from build123d import *

# Parameters (mm, degrees)
SKETCH_2_W                    = 37.5
SKETCH_2_H                    = 19
EXTRUDE_1_DEPTH               = 1.6
SKETCH_3_W                    = 23
SKETCH_3_H                    = 13.4
EXTRUDE_2_DEPTH               = 10.4
FILLET_1_R                    = 2
SKETCH_4_W                    = 4
SKETCH_4_H                    = 3
CUT_EXTRUDE_1_DEPTH           = 1.6
FILLET_2_R                    = 1.5
SKETCH_5_R                    = 1.5
CUT_EXTRUDE_2_DEPTH           = 5
SKETCH_6_W                    = 8
SKETCH_6_H                    = 6
CUT_EXTRUDE_3_DEPTH           = 1
CUT_EXTRUDE_3_DRAFT           = -57
CUT_EXTRUDE_3_PROFILE_2_DEPTH = 1
CUT_EXTRUDE_3_PROFILE_2_DRAFT = -57
FILLET_3_R                    = 5.5
SKETCH_7_W                    = 8
SKETCH_7_H                    = 7
EXTRUDE_3_DEPTH               = 1
SKETCH_8_W                    = 8
SKETCH_8_H                    = 3.15
SKETCH_8_H_2                  = 3.13772234
EXTRUDE_4_DEPTH               = 1
FILLET_4_R                    = 2
SKETCH_9_W                    = 3
SKETCH_9_H                    = 0.2
EXTRUDE_5_DEPTH               = 2
SKETCH_10_W                   = 3
SKETCH_10_H                   = 7
EXTRUDE_6_DEPTH               = 0.2
SKETCH_11_W                   = 1.5
SKETCH_11_H                   = 3
CUT_EXTRUDE_4_DEPTH           = 0.2
FILLET_5_R                    = 0.75


# Some blends are built 0.0001 mm under size
with BuildPart() as part:
    # Эскиз2 → Бобышка-Вытянуть1 (new body)
    with BuildSketch(Plane.XY):
        Rectangle(SKETCH_2_W, SKETCH_2_H)
    extrude(amount=EXTRUDE_1_DEPTH)

    # Эскиз3 → Бобышка-Вытянуть2 (add)
    with BuildSketch(Plane.XY.offset(1.6)):
        Rectangle(SKETCH_3_W, SKETCH_3_H)
    extrude(amount=EXTRUDE_2_DEPTH)

    # Скругление1
    fillet_1_edges = [part.edges().sort_by_distance(p)[0] for p in [
        (-18.75, 9.5, 0.8),
        (18.75, 9.5, 0.8),
        (18.75, -9.5, 0.8),
        (-18.75, -9.5, 0.8),
    ]]
    fillet(fillet_1_edges, radius=FILLET_1_R)

    # Эскиз4 → Вырез-Вытянуть1 (cut)
    with BuildSketch(Plane.XY.offset(1.6)):
        with Locations((14.75, 0)):
            Rectangle(SKETCH_4_W, SKETCH_4_H)
        with Locations((-14.75, 0)):
            Rectangle(SKETCH_4_W, SKETCH_4_H)
    extrude(amount=-CUT_EXTRUDE_1_DEPTH, mode=Mode.SUBTRACT)

    # Скругление2
    fillet_2_edges = [part.edges().sort_by_distance(p)[0] for p in [
        (-16.75, 1.5, 0.8),
        (-12.75, 1.5, 0.8),
        (16.75, 1.5, 0.8),
        (16.75, -1.5, 0.8),
        (-12.75, -1.5, 0.8),
        (-16.75, -1.5, 0.8),
        (12.75, -1.5, 0.8),
        (12.75, 1.5, 0.8),
    ]]
    fillet(fillet_2_edges, radius=FILLET_2_R - 0.0001)  # a hair under: the kernel refuses the full size

    # Эскиз5 → Вырез-Вытянуть2 (cut)
    with BuildSketch(Plane.XY.offset(12)):
        with Locations((-7.1, 2.7)):
            Circle(SKETCH_5_R)
        with Locations((7.1, 2.7)):
            Circle(SKETCH_5_R)
    extrude(amount=-CUT_EXTRUDE_2_DEPTH, mode=Mode.SUBTRACT)


with BuildPart() as cut_extrude_3_tool:
    # Эскиз6 → Вырез-Вытянуть3 (with draft: the straight prism first)
    with BuildSketch(Plane.XY.offset(12)):
        with Locations((-7.1, 2.7)):
            Rectangle(SKETCH_6_W, SKETCH_6_H)
    extrude(amount=-CUT_EXTRUDE_3_DEPTH)
    # Вырез-Вытянуть3: the draft: its side faces are tilted about the plane it starts from
    cut_extrude_3_sides = [cut_extrude_3_tool.faces().sort_by_distance(p)[0] for p in [
        (-11.1, 2.7, 11.5),
        (-7.1, -0.3, 11.5),
        (-3.1, 2.7, 11.5),
        (-7.1, 5.7, 11.5),
    ]]
    draft(cut_extrude_3_sides, Plane.XY.offset(12), CUT_EXTRUDE_3_DRAFT)


with BuildPart() as part_1:
    add(part.part)

    # Вырез-Вытянуть3: cut by cut_extrude_3_tool
    add(cut_extrude_3_tool.part, mode=Mode.SUBTRACT)


with BuildPart() as cut_extrude_3_profile_2_tool:
    # Эскиз6 → Вырез-Вытянуть3 profile 2 (with draft: the straight prism first)
    with BuildSketch(Plane.XY.offset(12)):
        with Locations((7.1, 2.7)):
            Rectangle(SKETCH_6_W, SKETCH_6_H)
    extrude(amount=-CUT_EXTRUDE_3_PROFILE_2_DEPTH)
    # Вырез-Вытянуть3 profile 2: the draft: its side faces are tilted about the plane it starts from
    cut_extrude_3_profile_2_sides = [cut_extrude_3_profile_2_tool.faces().sort_by_distance(p)[0] for p in [
        (3.1, 2.7, 11.5),
        (7.1, -0.3, 11.5),
        (11.1, 2.7, 11.5),
        (7.1, 5.7, 11.5),
    ]]
    draft(cut_extrude_3_profile_2_sides, Plane.XY.offset(12), CUT_EXTRUDE_3_PROFILE_2_DRAFT)


with BuildPart() as part_2:
    add(part_1.part)

    # Вырез-Вытянуть3 profile 2: cut by cut_extrude_3_profile_2_tool
    add(cut_extrude_3_profile_2_tool.part, mode=Mode.SUBTRACT)

    # Скругление3
    fillet_3_edges = [part_2.edges().sort_by_distance(p)[0] for p in [
        (0, -6.7, 12),
    ]]
    fillet(fillet_3_edges, radius=FILLET_3_R)

    # Эскиз7 → Бобышка-Вытянуть3 (add)
    with BuildSketch(Plane.XY.offset(12)):
        with Locations((-7.1, -4)):
            Rectangle(SKETCH_7_W, SKETCH_7_H)
        with Locations((7.1, -4)):
            Rectangle(SKETCH_7_W, SKETCH_7_H)
    extrude(amount=-EXTRUDE_3_DEPTH)

    # Эскиз8 → Бобышка-Вытянуть4 (add)
    with BuildSketch(Plane.XY.offset(12)):
        with Locations((-7.1, -5.925)):
            Rectangle(SKETCH_8_W, SKETCH_8_H)
        with Locations((7.1, -5.93113883)):
            Rectangle(SKETCH_8_W, SKETCH_8_H_2)
    extrude(amount=EXTRUDE_4_DEPTH)

    # Фаска1
    # the kernel refuses this chamfer: 3 mm, written as the material it adds along each edge
    with BuildSketch(Plane(origin=(-3.1, -4.35, 12), x_dir=(0, 0.9996219169112968, -0.027495876610586202), z_dir=(-1, 0, 0))) as chamfer_1_piece_1_section:
        with BuildLine():
            Line((3.086019586, 0), (-0.169641465, -3.081353381))
            Line((-0.169641465, -3.081353381), (-0.22961878, -3.079703628))
            ThreePointArc((-0.22961878, -3.079703628), (-0.102387681, -1.540193489), (-0.059977315, 0.001649753))
            Line((-0.059977315, 0.001649753), (0.001649753, 0.059977315))
            ThreePointArc((0.001649753, 0.059977315), (1.543492994, 0.017566949), (3.087669338, 0.059977315))
            Line((3.087669338, 0.059977315), (3.086019586, 0))
        make_face()
    chamfer_1_piece_1 = extrude(amount=8, mode=Mode.PRIVATE)
    chamfer_1_piece_1 = split(chamfer_1_piece_1, bisect_by=Plane(origin=(-7.1, -3.063879333, 13), z_dir=(0, 0, -1)), keep=Keep.TOP, mode=Mode.PRIVATE)
    add(chamfer_1_piece_1)
    with BuildSketch(Plane(origin=(11.1, -4.36227766, 12), x_dir=(0, 0.9996219169112968, -0.027495876610586202), z_dir=(-1, 0, 0))) as chamfer_1_piece_2_section:
        with BuildLine():
            Line((3.086019586, 0), (-0.169641465, -3.081353381))
            Line((-0.169641465, -3.081353381), (-0.22961878, -3.079703628))
            ThreePointArc((-0.22961878, -3.079703628), (-0.102387681, -1.540193489), (-0.059977315, 0.001649753))
            Line((-0.059977315, 0.001649753), (0.001649753, 0.059977315))
            ThreePointArc((0.001649753, 0.059977315), (1.543492994, 0.017566949), (3.087669338, 0.059977315))
            Line((3.087669338, 0.059977315), (3.086019586, 0))
        make_face()
    chamfer_1_piece_2 = extrude(amount=8, mode=Mode.PRIVATE)
    chamfer_1_piece_2 = split(chamfer_1_piece_2, bisect_by=Plane(origin=(7.1, -3.076156993, 13), z_dir=(0, 0, -1)), keep=Keep.TOP, mode=Mode.PRIVATE)
    add(chamfer_1_piece_2)

    # Скругление4
    # the kernel refuses this fillet: 2 mm, written as the material it adds along each edge
    with BuildSketch(Plane(origin=(5.017202419, -4.36227766, 11), x_dir=(0, -0.6120158801433927, -0.7908454731819031), z_dir=(-1, 0, 0))) as fillet_4_piece_1_section:
        with BuildLine():
            CenterArc((3.837222962, 1.910888885), FILLET_4_R, 163.424275541, 89.407933075)
            Line((1.920335899, 2.481453509), (1.881998158, 2.492864801))
            ThreePointArc((1.881998158, 2.492864801), (0.928534131, 1.265207389), (-0.031633819, 0.024480635))
            Line((-0.031633819, 0.024480635), (0.01180684, -0.038217778))
            ThreePointArc((0.01180684, -0.038217778), (1.623440484, 0.205055567), (3.235074128, -0.038217778))
            Line((3.235074128, -0.038217778), (3.246880968, 0))
        make_face()
    fillet_4_piece_1 = extrude(amount=16.117202419, mode=Mode.PRIVATE)
    fillet_4_piece_1 = split(fillet_4_piece_1, bisect_by=Plane(origin=(3.1, -5.888894845, 10.384505844), z_dir=(1, 0, 0)), keep=Keep.TOP, mode=Mode.PRIVATE)
    add(fillet_4_piece_1)
    with BuildSketch(Plane(origin=(-3.1, -4.36227766, 11), x_dir=(0, -0.6120158801433927, -0.7908454731819031), z_dir=(-1, 0, 0))) as fillet_4_piece_2:
        with BuildLine():
            CenterArc((3.837222962, 1.910888885), FILLET_4_R, 163.424275541, 89.407933075)
            Line((1.920335899, 2.481453509), (1.881998158, 2.492864801))
            ThreePointArc((1.881998158, 2.492864801), (0.928534131, 1.265207389), (-0.031633819, 0.024480635))
            Line((-0.031633819, 0.024480635), (0.01180684, -0.038217778))
            ThreePointArc((0.01180684, -0.038217778), (1.623440484, 0.205055567), (3.235074128, -0.038217778))
            Line((3.235074128, -0.038217778), (3.246880968, 0))
        make_face()
    extrude(amount=8)
    with BuildSketch(Plane(origin=(11.1, -4.36227766, 11), x_dir=(0, -1, 0), z_dir=(-1, 0, 0))) as fillet_4_piece_3:
        with BuildLine():
            CenterArc((3.859659213, -1.865156066), FILLET_4_R, 111.159682929, 89.407933075)
            Line((1.987142713, -2.567781115), (1.949692383, -2.581833616))
            ThreePointArc((1.949692383, -2.581833616), (1.155738623, -1.158393294), (-0.022998383, -0.032727273))
            Line((-0.022998383, -0.032727273), (0, 0.04))
            ThreePointArc((0, 0.04), (1.56886117, 0.04), (3.123283602, 0.037303121))
            Line((3.123283602, 0.037303121), (3.13772234, 0))
        make_face()
    extrude(amount=8)
    with BuildSketch(Plane(origin=(11.1, -4.36227766, 11), x_dir=(0, -1, 0), z_dir=(-1, 0, 0))) as fillet_4_piece_4_section:
        with BuildLine():
            CenterArc((3.859659213, -1.865156066), FILLET_4_R, 111.159682929, 89.407933075)
            Line((1.987142713, -2.567781115), (1.949692383, -2.581833616))
            ThreePointArc((1.949692383, -2.581833616), (1.155738623, -1.158393294), (-0.022998383, -0.032727273))
            Line((-0.022998383, -0.032727273), (0, 0.04))
            ThreePointArc((0, 0.04), (1.56886117, 0.04), (3.123283602, 0.037303121))
            Line((3.123283602, 0.037303121), (3.13772234, 0))
        make_face()
    fillet_4_piece_4 = extrude(amount=16.117202419, mode=Mode.PRIVATE)
    fillet_4_piece_4 = split(fillet_4_piece_4, bisect_by=Plane(origin=(-3.1, -5.888894845, 10.384505844), z_dir=(-1, 0, 0)), keep=Keep.TOP, mode=Mode.PRIVATE)
    add(fillet_4_piece_4)

    # Эскиз9 → Бобышка-Вытянуть5 (add)
    with BuildSketch(Plane(origin=(0, 0, 0), x_dir=(-1, 0, 0), z_dir=(0, 0, -1))):
        with Locations((-6.25, 5.4)):
            Rectangle(SKETCH_9_W, SKETCH_9_H)
        with Locations((6.25, 5.4)):
            Rectangle(SKETCH_9_W, SKETCH_9_H)
    extrude(amount=EXTRUDE_5_DEPTH)

    # Эскиз10 → Бобышка-Вытянуть6 (add)
    with BuildSketch(Plane(origin=(0, 0, -2), x_dir=(-1, 0, 0), z_dir=(0, 0, -1))):
        with Locations((-6.25, 2)):
            Rectangle(SKETCH_10_W, SKETCH_10_H)
        with Locations((6.25, 2)):
            Rectangle(SKETCH_10_W, SKETCH_10_H)
    extrude(amount=EXTRUDE_6_DEPTH)

    # Эскиз11 → Вырез-Вытянуть4 (cut)
    with BuildSketch(Plane(origin=(0, 0, -2.2), x_dir=(-1, 0, 0), z_dir=(0, 0, -1))):
        with Locations((-6.25, 0.75)):
            Rectangle(SKETCH_11_W, SKETCH_11_H)
        with Locations((6.25, 0.75)):
            Rectangle(SKETCH_11_W, SKETCH_11_H)
    extrude(amount=-CUT_EXTRUDE_4_DEPTH, mode=Mode.SUBTRACT)

    # Скругление5
    fillet_5_edges = [part_2.edges().sort_by_distance(p)[0] for p in [
        (-7, 2.25, -2.1),
        (-7, -0.75, -2.1),
        (5.5, -0.75, -2.1),
        (7, -0.75, -2.1),
        (-5.5, -0.75, -2.1),
        (-5.5, 2.25, -2.1),
        (4.75, -1.5, -2.1),
        (7, 2.25, -2.1),
        (7.75, -1.5, -2.1),
        (5.5, 2.25, -2.1),
        (-7.75, -1.5, -2.1),
        (-4.75, -1.5, -2.1),
    ]]
    fillet(fillet_5_edges, radius=FILLET_5_R - 0.0001)  # a hair under: the kernel refuses the full size


solid = part_2.part
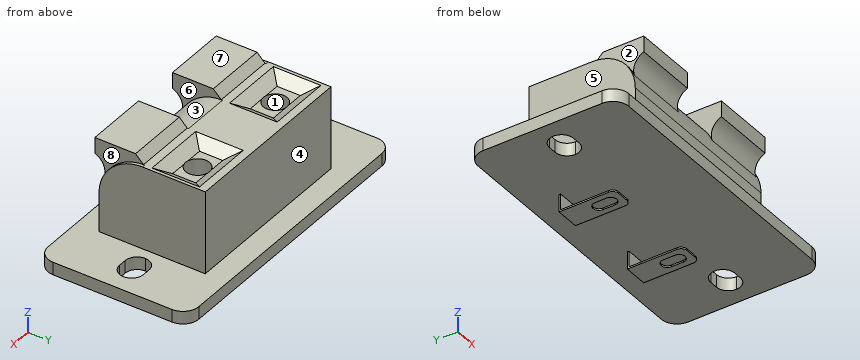
The listing builds one solid part. Answer for the finished solid, in the listing's coordinates (mm). Face numbers are marked on the shaded views. A direction names the side the tool comes from. Give positions to 0.01 mm unless a question says otherwise; leave off trailing zeros. Write each loop counter-clockwise with the first axis right and the second up, starting at its lowest first coordinate (ties: lowest second). Pieces come first, ordered by that corner, then holes. Notation, with made-up numbers: (63.5, -30) - (91.5, -30) arc R23 ccw to (91.5, -8) - close; hole circle Ø5 at (80.5, 3.5). An arc over 180 degrees is marked (long way). One line per question, with ' | ' between items. Start each with the question number.
1. Determine the mould class of the marked faces 5, 6, 7 and 8 for opening direction X: +X half, -X half, draft (parallel to the pull), parting line (faces both ways), or undercut.
2. Section B-B, the plane x = 16 is taken. Determine the outline of the cut face in (y, z), then the cut area to 3 significant figures.
3. Straight lines are drawn through the part: line 1 (Y direction, x = -7.1, z = 8.85); line 2 (X direction, y = -6, z = 9.25); line 3 (X direction, y = 1.25, z = 1.5). For each, find the intervals that lie inside material, in ascending order.
4. For the marked faces 1, 2, 3 and 4, determine the directions among +Z, -Z, +X, -X, +Y, -Y from which every point of the face is accessible in a straight line to the end or side of a thin tool.
5. Section C-C, the plane z = 10 is taken. Determine the outline of the cut face in (x, y).
6. Given P1, Ø1.8, axis at y = 2.5, z = -1.5, coming from the -X side; P2, Ø1.5, axis at x = 9.5, z = 9, coming from the +Y side; P3, Ø5, axis at y = -3, z = 11, coming from the +X side, each flat-ended and moving along its own axis, determine where each tip first touches the part or whether it passes through.
7. Section D-D, the plane x = 4 is taken. Determine the outline of the cut face in (y, z).
8. Section A-A, the plane y = 2.7 is taken. Count the separate pieces of the cut face and the enclosed holes in it, then the cut area to 3 significant figures.
Result:
1) face 5: -X half | face 6: undercut | face 7: draft | face 8: +X half
2) outline: (-9.5, 0) - (-1.3, 0) - (-1.3, 1.6) - (-9.5, 1.6) - close; (1.3, 0) - (9.5, 0) - (9.5, 1.6) - (1.3, 1.6) - close | area: 26.2 mm2
3) line 1: y = -6.24 to 1.2, 4.2 to 6.7 | line 2: x = -11.1 to -3.1, 3.1 to 11.1 | line 3: x = -18.75 to -16.08, -13.42 to 13.42, 16.08 to 18.75
4) face 1: +Z | face 2: +Z, -X, -Y | face 3: -Y | face 4: +Z, +X, -X, +Y
5) outline: (-11.5, -5.44) - (-11.1, -5.44) - (-11.1, -6.42) - (-3.1, -6.42) - (-3.1, -5.44) - (3.1, -5.44) - (3.1, -6.42) - (11.1, -6.42) - (11.1, -5.44) - (11.5, -5.44) - (11.5, 6.7) - (-11.5, 6.7) - close; hole circle Ø3 at (-7.1, 2.7); hole circle Ø3 at (7.1, 2.7)
6) P1: stops at x = -7.75 | P2: stops at y = 6.7 | P3: stops at x = 11.5
7) outline: (-9.5, 0) - (9.5, 0) - (9.5, 1.6) - (6.7, 1.6) - (6.7, 12) - (5.7, 12) - (4.8, 11.42) - (0.6, 11.42) - (-0.3, 12) - (-1.36, 12) - (-2.36, 13) - (-7.5, 13) - (-7.5, 11) arc R2 cw to (-6.35, 8.43) arc R5.5 ccw to (-6.7, 6.5) - (-6.7, 1.6) - (-9.5, 1.6) - close
8) separate pieces: 3 | enclosed holes: 0 | area: 263 mm2
